Design review of the part built by this model. Coordinates are the model's own, in mm. Coordinates: 2 decimals unless noted, no trailing zeros. Loops run counter-clockwise (first coordinate to the right, second up) from the corner with the lowest first, then second, coordinate; pieces in that order, holes last. Notation, with made-up numbers: (50, 29.25) -> (100, 29.25) arc R14 cw to (100, 38.25) -> close; hole circle Ø4 at (15, 78.5). An arc over 180 degrees is marked (long way). Use a Markdown table: item, result. Add a question column.
Q1. For probe 1 along Z at (x, y) = (-440, 2.8); probe 2 along Y at (x, z) = (-227.5, 2); probe 3 along X at (y, z) = (1.25, 46), list the stretches that pass through material, from the lowest coordinate up.
Q2. Clearance check with flat-ended pins moving along their axes: pin 1 Ø5.5 at (x, y) = (318.5, 14.7) entering from +Z; pin 2 Ø9.5 at (x, y) = (-318.5, 14.7) entering from +Z; pin 3 Ø5 at (x, y) = (-187, 2.5) entering from +Z; pin 4 Ø5 at (x, z) = (-346.5, 28.5) entering from +Y. State where each tip first meets the part, or that it passes through.
Q3. Take a section at B-B on z = 21. Write out the cut boundary in (x, y), plus the area to 3 significant figures.
Q4. Take a section at A-A on x = -298. Write out the cut boundary in (y, z).
from build123d import *

# Parameters (mm, degrees)
PAD_DEPTH         = 460
POCKET_DEPTH      = 26.001
POCKET_DEPTH_BACK = 0.001
SKETCH002_R       = 3
HOLE_DEPTH        = 25
SKETCH003_R       = 3.25
POCKET001_DEPTH   = 4.701


with BuildPart() as part:
    # Sketch → Pad (new body, symmetric)
    with BuildSketch(Plane.YZ):
        Polygon((0, 60), (4.7, 60), (4.7, 4.7), (26, 4.7), (26, 0), (0, 0), align=None)
    extrude(amount=PAD_DEPTH, both=True)

    # Sketch001 (on Face3 of Pad) → Pocket (cut, two sides)
    with BuildSketch(Plane(origin=(0, 0, 0), x_dir=(0, 0, -1), z_dir=(0, -1, 0))) as pocket_sk:
        with BuildLine():
            Line((-70, -427.5), (-36, -427.5))
            ThreePointArc((-36, -427.5), (-31.757359, -425.742641), (-30, -421.5))
            Line((-30, -421.5), (-30, 421.5))
            ThreePointArc((-30, 421.5), (-31.757359, 425.742641), (-36, 427.5))
            Line((-36, 427.5), (-70, 427.5))
            Line((-70, 427.5), (-70, -427.5))
        make_face()
    extrude(amount=-POCKET_DEPTH, mode=Mode.SUBTRACT)
    extrude(pocket_sk.sketch, amount=POCKET_DEPTH_BACK, mode=Mode.SUBTRACT)

    # Sketch002 (on Face2 of Pocket) → Hole (cut)
    with BuildSketch(Plane(origin=(0, 0, 4.7), x_dir=(0, -1, 0), z_dir=(0, 0, 1))):
        with Locations((-14.7, 455)):
            Circle(SKETCH002_R)
        with Locations((-14.7, 409.5)):
            Circle(SKETCH002_R)
        with Locations((-14.7, 364)):
            Circle(SKETCH002_R)
        with Locations((-14.7, 318.5)):
            Circle(SKETCH002_R)
        with Locations((-14.7, 273)):
            Circle(SKETCH002_R)
        with Locations((-14.7, 227.5)):
            Circle(SKETCH002_R)
        with Locations((-14.7, 182)):
            Circle(SKETCH002_R)
        with Locations((-14.7, 136.5)):
            Circle(SKETCH002_R)
        with Locations((-14.7, 91)):
            Circle(SKETCH002_R)
        with Locations((-14.7, 45.5)):
            Circle(SKETCH002_R)
        with Locations((-14.7, 0)):
            Circle(SKETCH002_R)
        with Locations((-14.7, -45.5)):
            Circle(SKETCH002_R)
        with Locations((-14.7, -91)):
            Circle(SKETCH002_R)
        with Locations((-14.7, -136.5)):
            Circle(SKETCH002_R)
        with Locations((-14.7, -182)):
            Circle(SKETCH002_R)
        with Locations((-14.7, -227.5)):
            Circle(SKETCH002_R)
        with Locations((-14.7, -273)):
            Circle(SKETCH002_R)
        with Locations((-14.7, -318.5)):
            Circle(SKETCH002_R)
        with Locations((-14.7, -364)):
            Circle(SKETCH002_R)
        with Locations((-14.7, -409.5)):
            Circle(SKETCH002_R)
        with Locations((-14.7, -455)):
            Circle(SKETCH002_R)
    extrude(amount=-HOLE_DEPTH, mode=Mode.SUBTRACT)

    # Sketch003 (on Face6 of Hole) → Pocket001 (cut, through all)
    with BuildSketch(Plane.ZX.offset(4.7)):
        with Locations((37.3, -440)):
            Circle(SKETCH003_R)
        with Locations((51.3, -440)):
            Circle(SKETCH003_R)
        with Locations((37.3, 440)):
            Circle(SKETCH003_R)
        with Locations((51.3, 440)):
            Circle(SKETCH003_R)
        with BuildLine():
            ThreePointArc((57, -437.75), (56, -436.75), (55, -437.75))
            Line((55, -437.75), (55, -442.25))
            ThreePointArc((55, -442.25), (56, -443.25), (57, -442.25))
            Line((57, -437.75), (57, -442.25))
        make_face()
        with BuildLine():
            Line((57, 437.75), (57, 442.25))
            ThreePointArc((59, 442.25), (58, 443.25), (57, 442.25))
            Line((59, 442.25), (59, 437.75))
            ThreePointArc((57, 437.75), (58, 436.75), (59, 437.75))
        make_face()
    extrude(amount=-POCKET001_DEPTH, mode=Mode.SUBTRACT)


solid = part.part
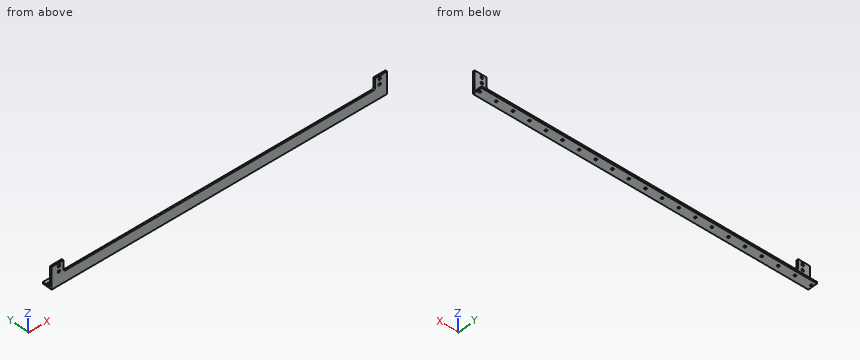
Answer list:
| question | item | result |
|---|---|---|
| 1 | probe 1 | 0 to 34.05, 40.55 to 48.05, 54.55 to 55, 57 to 60 |
| 1 | probe 2 | 0 to 11.7, 17.7 to 26 |
| 1 | probe 3 | -460 to -427.5, 427.5 to 460 |
| 2 | pin 1 | through |
| 2 | pin 2 | z = 4.7 |
| 2 | pin 3 | z = 30 |
| 2 | pin 4 | y = 4.7 |
| 3 | outline | (-460, 0) -> (460, 0) -> (460, 4.7) -> (-460, 4.7) -> close |
| 3 | area | 4,320 mm² |
| 4 | outline | (0, 0) -> (26, 0) -> (26, 4.7) -> (4.7, 4.7) -> (4.7, 30) -> (0, 30) -> close |
